Read the model definition and answer for the solid it produces. Units are mm, in the model's axes. Face numbers are marked on the shaded views. A direction names the side the tool comes from. Coordinates: 2 decimals unless noted, no trailing zeros. Write each loop counter-clockwise with the first axis right and the second up, starting at its lowest first coordinate (ties: lowest second). Pieces come first, ordered by that corner, then holes.
(1) Determine the mould class of the marked faces 3, 4 and 5 for opening direction Z: pulls with the +Z half, pulls with the -Z half, needs draft (parallel to the pull), parting line crosses it, or undercut.
(2) The part is cut by section A-A, the plane z = 16. Determine the outline of the cut face in (x, y).
(3) Straight lines are drawn through the part: line 1 along Y through (x, z) = (7, 20.5); line 2 along X through (y, z) = (2.5, 15); line 3 along Z through (x, y) = (18, 0.7). For each, find the intervals that lie inside material, in ascending order.
(4) The part is cut by section D-D, the plane z = 21.5. Determine the outline of the cut face in (x, y), and give its area (3 significant figures).
(5) Given pin 1 (0.6 mm diameter, centred on y = -1.5, z = 26, fed in from +X); pin 2 (2 mm diameter, centred on x = 30, y = 0.5, fed in from -Z); pin 3 (1.6 mm diameter, centred on x = 30.5, y = -1, fed in from +Z); pin 4 (1.6 mm diameter, centred on x = 30, z = 26.5, fed in from -Y), each flat-ended and moving along its own axis, determine where each tip first touches the part or whether it passes through.
(6) The part is cut by section B-B, the plane y = 1.55. Determine the outline of the cut face in (x, z).
(7) The part is cut by section C-C, the plane x = 13. Determine the outline of the cut face in (y, z), and give its area (3 significant figures).
(8) Which of the six approach directions +Z, -Z, +X, -X, +Y, -Y give full straight-line access (tool end or side, diameter ignored) to the marked faces 1 and 2?
```python
from build123d import *

# Parameters (mm, degrees)
SKETCH1_W          = 31.2
SKETCH1_H          = 32.2
BODY_DEPTH         = 4
SKETCH2_W          = 2
SKETCH2_H          = 2
FEMALE_TABS_DEPTH  = 2
SKETCH3_W          = 2
SKETCH3_H          = 2
MALE_TABS_DEPTH    = 2
SKETCH4_W          = 5
SKETCH4_H          = 5
CUT_EXTRUDE2_DEPTH = 4
CUT_EXTRUDE2_DRAFT = -10


with BuildPart() as part:
    # Sketch1 → Body (new body)
    with BuildSketch(Plane(origin=(0, 0, 0), x_dir=(1, 0, 0), z_dir=(0, 1, 0))):
        with Locations((15.6, -16.1)):
            Rectangle(SKETCH1_W, SKETCH1_H)
    extrude(amount=BODY_DEPTH)

    # Sketch2 → Female Tabs (cut)
    with BuildSketch(Plane(origin=(0, 0, 0), x_dir=(-1, 0, 0), z_dir=(0, -1, 0))):
        with Locations((-1, -4.9)):
            Rectangle(SKETCH2_W, SKETCH2_H)
        with Locations((-30.2, -26.2)):
            Rectangle(SKETCH2_W, SKETCH2_H)
    extrude(amount=-FEMALE_TABS_DEPTH, mode=Mode.SUBTRACT)

    # Sketch3 → Male Tabs (add)
    with BuildSketch(Plane(origin=(0, 0, 0), x_dir=(-1, 0, 0), z_dir=(0, -1, 0))):
        with Locations((-1, -26.2)):
            Rectangle(SKETCH3_W, SKETCH3_H)
        with Locations((-30.2, -4.9)):
            Rectangle(SKETCH3_W, SKETCH3_H)
    extrude(amount=MALE_TABS_DEPTH)


with BuildPart() as cut_extrude2_tool:
    # Sketch4 → Cut-Extrude2 (with draft: the straight prism first)
    with BuildSketch(Plane(origin=(0, 4, 0), x_dir=(1, 0, 0), z_dir=(0, 1, 0))):
        with Locations((16.2, -17.2)):
            Rectangle(SKETCH4_W, SKETCH4_H)
    extrude(amount=-CUT_EXTRUDE2_DEPTH)
    # Cut-Extrude2: the draft: its side faces are tilted about the plane it starts from
    cut_extrude2_sides = [cut_extrude2_tool.faces().sort_by_distance(p)[0] for p in [
        (18.7, 2, 17.2),
        (16.2, 2, 14.7),
        (13.7, 2, 17.2),
        (16.2, 2, 19.7),
    ]]
    draft(cut_extrude2_sides, Plane(origin=(0, 4, 0), x_dir=(1, 0, 0), z_dir=(0, 1, 0)), CUT_EXTRUDE2_DRAFT)


with BuildPart() as part_1:
    add(part.part)

    # Cut-Extrude2: cut by cut_extrude2_tool
    add(cut_extrude2_tool.part, mode=Mode.SUBTRACT)


solid = part_1.part
```
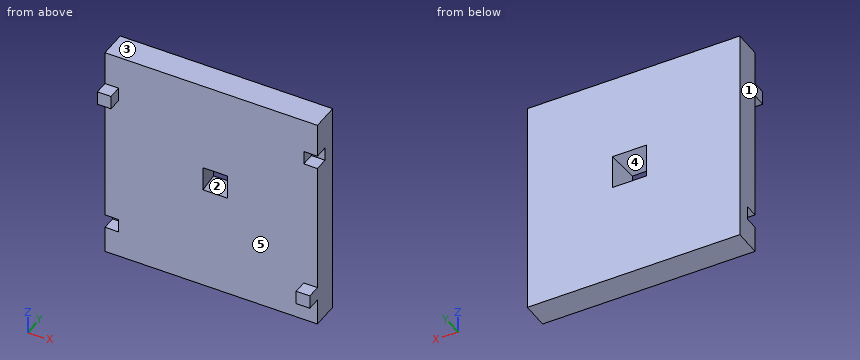
Computed:
1. face 3: pulls with the +Z half
1. face 4: undercut
1. face 5: needs draft
2. outline: (0, 0) - (14.41, 0) - (13.7, 4) - (0, 4) - close; (17.99, 0) - (31.2, 0) - (31.2, 4) - (18.7, 4) - close
3. line 1: y = 0 to 4
3. line 2: x = 0 to 13.96, 18.44 to 31.2
3. line 3: z = 0 to 15.28, 19.12 to 32.2
4. outline: (0, 0) - (31.2, 0) - (31.2, 4) - (0, 4) - close
4. area: 125 mm2
5. pin 1: stops at x = 2
5. pin 2: stops at z = 0
5. pin 3: stops at z = 5.9
5. pin 4: stops at y = 0
6. outline: (0, 0) - (31.2, 0) - (31.2, 25.2) - (29.2, 25.2) - (29.2, 27.2) - (31.2, 27.2) - (31.2, 32.2) - (0, 32.2) - (0, 5.9) - (2, 5.9) - (2, 3.9) - (0, 3.9) - close; hole (14.13, 15.13) - (18.27, 15.13) - (18.27, 19.27) - (14.13, 19.27) - close
7. outline: (0, 0) - (4, 0) - (4, 32.2) - (0, 32.2) - close
7. area: 129 mm2
8. face 1: +Z, -Z, -X, +Y, -Y
8. face 2: +Y
